from build123d import *

# Parameters (mm, degrees)
F1_DEPTH = 7.112
F2_DEPTH = 17.78
F4_DEPTH = 1.016
F5_DEPTH = 1.016


with BuildPart() as f1:
    # F0 (on Top) → F1 (new body)
    with BuildSketch(Plane.XY):
        with BuildLine():
            ThreePointArc((6.6260949281, -8.2945636224), (3.7152332811, 0), (6.6260949281, 8.2945636224))
            Line((6.6260949281, 8.2945636224), (-18.9858246595, 8.2945636224))
            Line((-18.9858246595, 8.2945636224), (-18.9858246595, -8.2945636224))
            Line((-18.9858246595, -8.2945636224), (6.6260949281, -8.2945636224))
        make_face()
    extrude(amount=F1_DEPTH)

    # F0 (on Top) → F2 (join)
    with BuildSketch(Plane.XY):
        with BuildLine():
            Line((6.6260949281, 8.2945636224), (9.6757363367, 8.2945636224))
            ThreePointArc((9.6757363367, 8.2945636224), (21.5388654762, 10.0781398953), (28.046251553, 0))
            ThreePointArc((28.046251553, 0), (21.5388654762, -10.0781398953), (9.6757363367, -8.2945636224))
            Line((9.6757363367, -8.2945636224), (6.6260949281, -8.2945636224))
            ThreePointArc((6.6260949281, -8.2945636224), (21.3836842093, -12.5243614328), (30.2616345138, 0))
            ThreePointArc((30.2616345138, 0), (21.3836842093, 12.5243614328), (6.6260949281, 8.2945636224))
        make_face()
        with BuildLine():
            ThreePointArc((9.6757363367, -8.2945636224), (5.930616242, 0), (9.6757363367, 8.2945636224))
            Line((9.6757363367, 8.2945636224), (6.6260949281, 8.2945636224))
            ThreePointArc((6.6260949281, 8.2945636224), (3.7152332811, 0), (6.6260949281, -8.2945636224))
            Line((6.6260949281, -8.2945636224), (9.6757363367, -8.2945636224))
        make_face()
    extrude(amount=F2_DEPTH)

    # F3 (on Front) → F4 (join)
    with BuildSketch(Plane.XZ):
        Polygon((-12.7892365647, 7.112), (5.8557423763, 7.112), (5.8557423763, 17.78), align=None)
    extrude(amount=F4_DEPTH)

    # F5 (add): a face of the model
    f5_faces = [f1.faces().sort_by_distance(p)[0] for p in [
        (-1.7862566675, 0, 10.2597587053),
    ]]
    extrude(f5_faces, amount=F5_DEPTH)


solid = f1.part
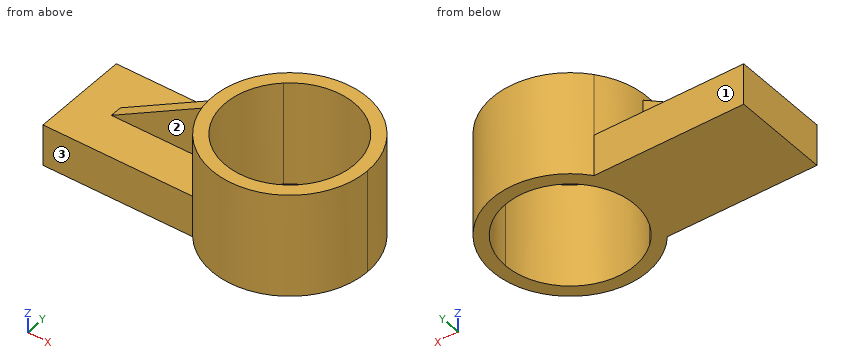
Source: CAD feature listing. Evaluate the final solid. Frame: model axes, mm. Face numbers are marked on the shaded views. A direction names the side the tool comes from. Round coordinates to 2 decimals unless told otherwise and drop trailing zeros. Loops run counter-clockwise (first coordinate to the right, second up) from the corner with the lowest first, then second, coordinate; pieces in that order, holes last. Notation, with made-up numbers: M 54.5,-13.5 L 75.5,-13.5 A24 cw 75.5,24.5 Z; hole C 55,51.25 d5. An arc over 180 degrees is marked long. Return JSON: item names as keys, results as strings. Group by question number.
1. Reachability of the marked faces 1, 2 and 3 from +Z, -Z, +X, -X, +Y, -Y: full face, straight path, thin tool, end or side. Return the list, or none.
2. Section query B-B on x = 22.5. Output: boundary loops of the cut face in (y, z).
3. Section query D-D on x = 2. Output: boundary loops of the cut face in (y, z).
4. Material intervals for line 1 along Y through (x, z) = (-5, 1); line 2 along Z through (x, y) = (-1, 5.25); line 3 along Y through (x, z) = (15.5, 1.25), sorted ascending. Write a range as from..to.
5. Section query A-A on y = -6. Output: boundary loops of the cut face in (x, z), and give its area (3 significant figures).
6. Section query C-C on z = 6. Output: boundary loops of the cut face in (x, y).
7. Pin query (flat end, axial travel): pin 1 (8 mm diameter, centred on x = 6, z = 7, fed in from -Y); pin 2 (10 mm diameter, centred on x = -12, y = -10.5, fed in from -Z); pin 3 (7.5 mm diameter, centred on x = -4, z = 10, fed in from +Y); pin 4 (8 mm diameter, centred on x = -4.5, z = 3.5, fed in from -Y). Return the tip coordinate at first contact, or that it passes through.
Checks:
{
 "1": {"face 1": "+Z, -Z, -X, +Y", "face 2": "+Z, -X, -Y", "face 3": "+Z, -Z, -X, -Y"},
 "2": {"outline": "M -12.07,0 L -9.59,0 L -9.59,17.78 L -12.07,17.78 Z; M 9.59,0 L 12.07,0 L 12.07,17.78 L 9.59,17.78 Z"},
 "3": {"outline": "M -8.29,0 L 8.29,0 L 8.29,7.11 L 1.02,7.11 L 1.02,15.57 L -1.02,15.57 L -1.02,7.11 L -8.29,7.11 Z"},
 "4": {"line 1": "y = -8.29..8.29", "line 2": "z = 0..7.11", "line 3": "y = -13.19..-10.96, 10.96..13.19"},
 "5": {"outline": "M -18.99,0 L 7.7,0 L 7.7,17.78 L 5.15,17.78 L 5.15,7.11 L -18.99,7.11 Z; M 26.28,0 L 28.83,0 L 28.83,17.78 L 26.28,17.78 Z", "area": "262 mm²"},
 "6": {"outline": "M -18.99,-8.29 L 6.63,-8.29 A13.27 ccw long 6.63,8.29 L -18.99,8.29 Z; hole C 16.99,0 d22.12"},
 "7": {"pin 1": "stops at y = -11.28", "pin 2": "stops at z = 0", "pin 3": "stops at y = 8.29", "pin 4": "stops at y = -8.29"}
}
